from build123d import *

# Parameters (mm, degrees)
BOSS_EXTRU_1_DEPTH      = 1
ESQUISSE2_W             = 5
ESQUISSE2_H             = 40.838750305
ESQUISSE2_H_2           = 45
BOSS_EXTRU_2_DEPTH      = 1
ESQUISSE3_W             = 125.749218941
ESQUISSE3_H             = 2
ESQUISSE3_W_2           = 13
BOSS_EXTRU_3_DEPTH      = 2
CHANFREIN1_SIZE         = 1.5
CHANFREIN2_SIZE         = 1
ENL_V_MAT_EXTRU_1_DEPTH = 339.434208864


with BuildPart() as part:
    # Esquisse1 → Boss.-Extru.1 (new body)
    with BuildSketch(Plane.XY):
        Polygon((-318.4, 56.6), (-203.4, 56.6), (-203.4, 1.6), (-14.350781059, 1.6), (-14.350781059, 107.438750305), (-318.4, 107.438750305), align=None)
    extrude(amount=-BOSS_EXTRU_1_DEPTH)

    # Esquisse2 → Boss.-Extru.2 (add)
    with BuildSketch(Plane(origin=(0, 0, -1), x_dir=(-1, 0, 0), z_dir=(0, 0, -1))):
        with Locations((318.421530381, 82.019375153)):
            Rectangle(ESQUISSE2_W, ESQUISSE2_H)
        with Locations((203.9, 29.1)):
            Rectangle(ESQUISSE2_W, ESQUISSE2_H_2)
    extrude(amount=BOSS_EXTRU_2_DEPTH)

    # Esquisse3 → Boss.-Extru.3 (add)
    with BuildSketch(Plane(origin=(0, 0, -1), x_dir=(-1, 0, 0), z_dir=(0, 0, -1))):
        with Locations((87.22539053, 57.6)):
            Rectangle(ESQUISSE3_W, ESQUISSE3_H)
        with Locations((87.22539053, 54)):
            Rectangle(ESQUISSE3_W, ESQUISSE3_H)
        with Locations((191.9, 57.6)):
            Rectangle(ESQUISSE3_W_2, ESQUISSE3_H)
        with Locations((191.9, 54)):
            Rectangle(ESQUISSE3_W_2, ESQUISSE3_H)
    extrude(amount=BOSS_EXTRU_3_DEPTH)

    # Chanfrein1
    chanfrein1_edges = [part.edges().sort_by_distance(p)[0] for p in [
        (-87.22539053, 58.6, -3),
        (-87.22539053, 53, -3),
        (-191.9, 58.6, -3),
        (-191.9, 53, -3),
    ]]
    chamfer(chanfrein1_edges, length=CHANFREIN1_SIZE)

    # Chanfrein2
    chanfrein2_edges = [part.edges().sort_by_distance(p)[0] for p in [
        (-201.4, 29.1, -1),
        (-315.921530381, 82.019375153, -1),
    ]]
    chamfer(chanfrein2_edges, length=CHANFREIN2_SIZE - 0.0001)  # a hair under: the kernel refuses the full size

    # Esquisse4 → Enlèv. mat.-Extru.1 (cut, through all)
    with BuildSketch(Plane(origin=(0, 0, -1), x_dir=(-1, 0, 0), z_dir=(0, 0, -1))):
        Polygon((90.245471521, 6.206378309), (85.245471521, 6.206378309), (99.094461568, 45.651267323), (104.094461568, 45.651267323), align=None)
        Polygon((94.094461568, 45.651267323), (80.245471521, 6.206378309), (75.245471521, 6.206378309), (89.094461568, 45.651267323), align=None)
        Polygon((84.094461568, 45.651267323), (70.245471521, 6.206378309), (65.245471521, 6.206378309), (79.094461568, 45.651267323), align=None)
        Polygon((74.094461568, 45.651267323), (60.245471521, 6.206378309), (55.245471521, 6.206378309), (69.094461568, 45.651267323), align=None)
        Polygon((64.094461568, 45.651267323), (50.245471521, 6.206378309), (45.245471521, 6.206378309), (59.094461568, 45.651267323), align=None)
        Polygon((54.094461568, 45.651267323), (40.245471521, 6.206378309), (35.245471521, 6.206378309), (49.094461568, 45.651267323), align=None)
    extrude(amount=-ENL_V_MAT_EXTRU_1_DEPTH, mode=Mode.SUBTRACT)


solid = part.part
Here's how the part is built. I have some questions about the finished solid (model axes, mm). A direction names the side the tool comes from. Coordinates: 2 decimals unless noted, no trailing zeros. Write each loop counter-clockwise with the first axis right and the second up, starting at its lowest first coordinate (ties: lowest second). Pieces come first, ordered by that corner, then holes.
Item 1: If I drill on line 1 (X direction, y = 54.5, z = -1.8); line 2 (Z direction, x = -261, y = 85); line 3 (X direction, y = 48, z = -0.15), over which ranges is the centre line in solid material (lowest first)?
Item 2: I want a section at B-B on x = -136. Write out the boundary of the cut face in (y, z).
Item 3: Will these pins go through, and if not, where does the flat tip stop? pin 1 (1.1 mm diameter, centred on x = -204, z = -1.5, fed in from -Y); pin 2 (0.8 mm diameter, centred on x = -320.5, y = 75, fed in from +Z); pin 3 (4 mm diameter, centred on x = -101.5, y = 75, fed in from -Z).
Item 4: I want a section at A-A on z = -2.5. Write out the boundary of the cut face in (x, y).
Item 5: On a 3-axis mill with a long thin cutter (end or side, diameter ignored), from which of +Z, -Z, +X, -X, +Y, -Y can I reach the whole of each face in a straight line? I mean faces 1 (the flat face through (-135, 67, 0)), 2 (the flat face through (-57.267, 26.205, -0.507)). Say none if no direction works.
Item 6: If we mould it in two halves opening along X, with no side actions, what happens to faces 3 (the flat face through (-47.267, 26.205, -0.507)), 4 (the flat face through (-204, 29, -2))? For each: +X half, -X half, draft (parallel to the pull), parting line (faces both ways), or undercut.
Item 7: I want a section at D-D on y = 12. Count the separate pieces of the cut face and the enclosed holes in it, and give its area (3 significant figures).
Findings below:
1. line 1: x = -198.4 to -185.4, -150.1 to -24.35
1. line 2: z = -1 to 0
1. line 3: x = -203.4 to -14.35
2. outline: (1.6, -1) - (53, -1) - (53, -1.5) - (54.5, -3) - (55, -3) - (55, -1) - (56.6, -1) - (56.6, -3) - (57.1, -3) - (58.6, -1.5) - (58.6, -1) - (107.44, -1) - (107.44, 0) - (1.6, 0) - close
3. pin 1: stops at y = 6.6
3. pin 2: stops at z = -1
3. pin 3: stops at z = -1
4. outline: (-198.4, 54) - (-185.4, 54) - (-185.4, 55) - (-198.4, 55) - close; (-198.4, 56.6) - (-185.4, 56.6) - (-185.4, 57.6) - (-198.4, 57.6) - close; (-150.1, 54) - (-24.35, 54) - (-24.35, 55) - (-150.1, 55) - close; (-150.1, 56.6) - (-24.35, 56.6) - (-24.35, 57.6) - (-150.1, 57.6) - close
5. face 1: +Z, +X, -X, +Y, -Y
5. face 2: +Z, -Z
6. face 3: undercut
6. face 4: draft
7. separate pieces: 7
7. enclosed holes: 0
7. area: 165 mm2
